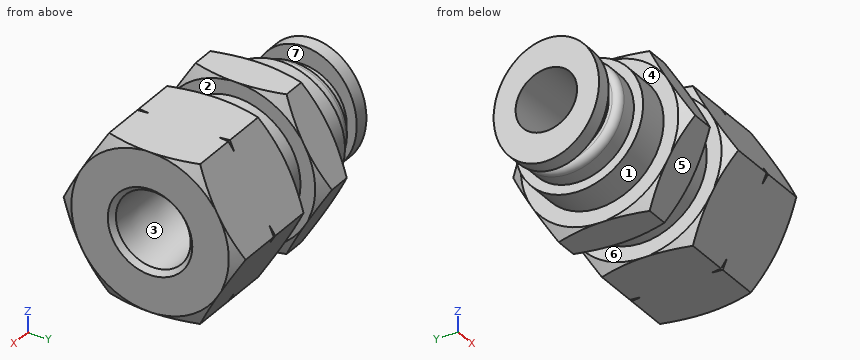
```python
from build123d import *

# Parameters (mm, degrees)
BOSS_EXTRUDE1_DEPTH = 13.49375
CHAMFER1_SIZE2      = 0.508
CHAMFER1_SIZE       = 0.525425432
SKETCH3_RX          = 6.50875
SKETCH3_RY          = 5.6769
SKETCH3_R           = 3.3147
BOSS_EXTRUDE2_DEPTH = 1.5875


with BuildPart() as part:
    # Sketch1 → Boss-Extrude1 (new body, symmetric)
    with BuildSketch(Plane(origin=(0, 0, 0), x_dir=(0, 0, -1), z_dir=(1, 0, 0))):
        Polygon((0, 9.796017487), (-8.4836, 4.898008744), (-8.4836, -4.898008744), (0, -9.796017487), (8.4836, -4.898008744), (8.4836, 4.898008744), align=None)
    extrude(amount=BOSS_EXTRUDE1_DEPTH, both=True)

    # Sketch2 → Cut-Revolve1 (revolve, cut)
    with BuildSketch(Plane.XY):
        Polygon((13.49375, 9.796017487), (13.49375, 8.4836), (12.73602541, 9.796017487), align=None)
        Polygon((3.17707459, 9.796017487), (-1.51337459, 9.796017487), (-0.75565, 8.4836), (-0.75565, 6.90245), (2.41935, 6.90245), (2.41935, 8.4836), align=None)
        Polygon((7.82043181, 9.796017487), (7.95655, 9.288017487), (8.09266819, 9.796017487), align=None)
        with BuildLine():
            Line((-3.94762541, 9.796017487), (-4.70535, 8.4836))
            Line((-4.70535, 8.4836), (-4.70535, 6.90245))
            Line((-4.70535, 6.90245), (-8.09625, 6.90245))
            Line((-8.09625, 6.90245), (-8.09625, 5.9055))
            Line((-8.09625, 5.9055), (-9.72185, 5.9055))
            ThreePointArc((-9.72185, 5.9055), (-10.260665367, 5.682315367), (-10.48385, 5.1435))
            Line((-10.48385, 5.1435), (-10.48385, 4.7625))
            Line((-10.48385, 4.7625), (-11.65225, 4.7625))
            Line((-11.65225, 4.7625), (-11.65225, 3.81))
            Line((-11.65225, 3.81), (-13.49375, 3.81))
            Line((-13.49375, 3.81), (-13.49375, 9.796017487))
            Line((-13.49375, 9.796017487), (-3.94762541, 9.796017487))
        make_face()
        Polygon((13.49375, 4.043670494), (4.19735, 3.74015), (3.497110726, 2.5273), (2.25425, 2.5273), (2.25425, 3.81), (-5.87375, 3.81), (-5.87375, 3.3147), (-13.49375, 3.3147), (-13.49375, 0), (13.49375, 0), align=None)
    revolve(axis=Axis((13.49375, 0, 0), (-1, 0, 0)), mode=Mode.SUBTRACT)

    # Chamfer1
    chamfer1_edges = [part.edges().sort_by_distance(p)[0] for p in [
        (13.49375, -4.043670494, 0),
    ]]
    chamfer(chamfer1_edges, length=CHAMFER1_SIZE, length2=CHAMFER1_SIZE2)

    # Sketch3 → Boss-Extrude2 (add)
    with BuildSketch(Plane.ZY.offset(13.49375)):
        with Locations(Location((0, 0), (0, 0, 180))):
            Ellipse(SKETCH3_RX, SKETCH3_RY)
        Circle(SKETCH3_R, mode=Mode.SUBTRACT)
    extrude(amount=-BOSS_EXTRUDE2_DEPTH)


solid = part.part
```
Work out the finished part from the listing and answer in its coordinate system (mm). Face numbers are marked on the shaded views. A direction names the side the tool comes from. Coordinates: 2 decimals unless noted, no trailing zeros. Loops run counter-clockwise (first coordinate to the right, second up) from the corner with the lowest first, then second, coordinate; pieces in that order, holes last. Notation, with made-up numbers: M 67,-39.5 L 79,-39.5 A16 ccw 79,-22.5 Z; hole C 83.25,-39.5 d9. An arc over 180 degrees is marked long. Use CSV: the item, a comma, the result in double quotes. Start each with the question number.
(1) Find section C-C, the plane x = 0.25. Give the vertices of the cut face in (y, z), then the cut area to 3 significant figures.
(2) Find section B-B, the plane x = 10.75. Give the vertices of the cut face in (y, z), then the cut area to 3 significant figures.
(3) Consider line 1 (Z direction, x = -9.75, y = 0); line 2 (X direction, y = 7.5, z = 0). Determine where each line is inside the solid, lowest interval first.
(4) For the marked faces 1, 2 and 3, determine the directions among +Z, -Z, +X, -X, +Y, -Y from which every point of the face is accessible in a straight line to the end or side of a thin tool.
(5) Find section A-A, the plane x = -3.25. Give the vertices of the cut face in (y, z).
(6) Given pin 1 Ø1.5 at (y, z) = (-0.5, 0) entering from -X; pin 2 Ø2.5 at (y, z) = (1, -1) entering from -X; pin 3 Ø7 at (y, z) = (0, 0) entering from +X; pin 4 Ø6 at (x, z) = (10.5, -2.5) entering from +Y, each flat-ended and moving along its own axis, determine where each tip first touches the part or whether it passes through.
(7) For a pull along X with two mould halves and no side action, classify the marked faces 4, 5, 6 and 7 as +X half, -X half, draft (parallel to the pull), parting line (faces both ways), or undercut.
Recorded:
1,outline,"C 0,0 d13.8; hole C 0,0 d7.62"
1,area,"104 mm^2"
2,outline,"M -9.8,0 L -4.9,-8.48 L 4.9,-8.48 L 9.8,0 L 4.9,8.48 L -4.9,8.48 Z; hole C 0,0 d7.91"
2,area,"200 mm^2"
3,line 1,"z = -5.9 to -3.31, 3.31 to 5.9"
3,line 2,"x = -4.71 to -0.76, 2.42 to 13.49"
4,face 1,"-X"
4,face 2,"none"
4,face 3,"+X"
5,outline,"M -9.8,0 L -4.9,-8.48 L 4.9,-8.48 L 9.8,0 L 4.9,8.48 L -4.9,8.48 Z; hole C 0,0 d7.62"
6,pin 1,"passes through"
6,pin 2,"stops at x = 2.25"
6,pin 3,"stops at x = 4.06"
6,pin 4,"stops at y = 9.8"
7,face 4,"-X half"
7,face 5,"draft"
7,face 6,"undercut"
7,face 7,"undercut"
